Geometry check sheet. Reference: the model listing, model coordinates, mm. Coordinates: 2 decimals unless noted, no trailing zeros. Write each loop counter-clockwise with the first axis right and the second up, starting at its lowest first coordinate (ties: lowest second). Pieces come first, ordered by that corner, then holes. Notation, with made-up numbers: (65, 30.5) -> (71, 30.5) arc R9 ccw to (71, 41.5) -> close; hole circle Ø1 at (-22, 69.25). An arc over 180 degrees is marked (long way). Answer as CSV lines item,"result".
```python
from build123d import *

# Parameters (mm, degrees)
F0_W     = 292.1
F0_H     = 50.8
F1_DEPTH = 12.7
F6_D     = 4.9784
F7_W     = 2.413
F7_H     = 2.8018399096
F8_DEPTH = 292.1


with BuildPart() as f1:
    # F0 (on Top) → F1 (new body)
    with BuildSketch(Plane.XY):
        with Locations((146.05, 25.4)):
            Rectangle(F0_W, F0_H)
    extrude(amount=-F1_DEPTH)

    # F6 (through all)
    with Locations(Plane.XY):
        with Locations((6.35, 40.64), (285.75, 40.64), (285.75, 10.16), (6.35, 10.16)):
            Hole(F6_D / 2)

    # F7 (on face) → F8 (cut, through all)
    with BuildSketch(Plane.YZ.offset(292.1)):
        Polygon((3.81, -3.81), (0, -3.81), (0, -5.4102), (2.413, -5.4102), (3.81, -5.4102), align=None)
        with Locations((1.2065, -6.8111199548)):
            Rectangle(F7_W, F7_H)
        Polygon((2.413, -8.2120399096), (0, -8.2120399096), (0, -12.7), (3.81, -12.7), (3.81, -8.2120399096), align=None)
        Polygon((50.8, -5.4102), (50.8, -3.81), (46.99, -3.81), (46.99, -5.4102), (48.387, -5.4102), align=None)
        with Locations((49.5935, -6.8111199548)):
            Rectangle(F7_W, F7_H)
        Polygon((46.99, -8.2120399096), (46.99, -12.7), (50.8, -12.7), (50.8, -8.2120399096), (48.387, -8.2120399096), align=None)
    extrude(amount=-F8_DEPTH, mode=Mode.SUBTRACT)


solid = f1.part
```
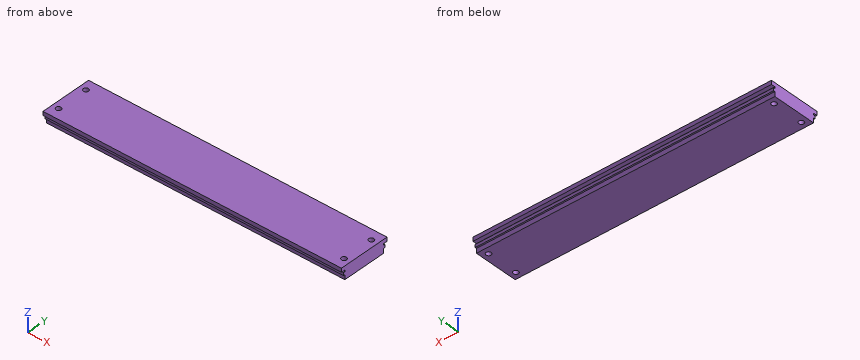
Item 1: Cross-section at B-B, the plane y = 40.64. Record the cut outline in (x, z), plus the area to 3 significant figures.
Responses:
outline,"(0, -12.7) -> (3.86, -12.7) -> (3.86, 0) -> (0, 0) -> close; (8.84, -12.7) -> (283.26, -12.7) -> (283.26, 0) -> (8.84, 0) -> close; (288.24, -12.7) -> (292.1, -12.7) -> (292.1, 0) -> (288.24, 0) -> close"
area,"3,580 mm2"
Item 2: Thickness scan on probe 1 along Y at (x, z) = (285.75, -10); probe 2 along Y at (x, z) = (285.75, -7); probe 3 along Y at (x, z) = (133, -8.75). Record the ranges inside material, lowest first.
Responses:
probe 1,"y = 3.81 to 7.67, 12.65 to 38.15, 43.13 to 46.99"
probe 2,"y = 2.41 to 7.67, 12.65 to 38.15, 43.13 to 48.39"
probe 3,"y = 3.81 to 46.99"
Item 3: Cross-section at C-C, the plane x = 285.75. Record the cut outline in (y, z).
Responses:
outline,"(0, -3.81) -> (3.81, -3.81) -> (3.81, -5.41) -> (2.41, -5.41) -> (2.41, -8.21) -> (3.81, -8.21) -> (3.81, -12.7) -> (7.67, -12.7) -> (7.67, 0) -> (0, 0) -> close; (12.65, -12.7) -> (38.15, -12.7) -> (38.15, 0) -> (12.65, 0) -> close; (43.13, -12.7) -> (46.99, -12.7) -> (46.99, -8.21) -> (48.39, -8.21) -> (48.39, -5.41) -> (46.99, -5.41) -> (46.99, -3.81) -> (50.8, -3.81) -> (50.8, 0) -> (43.13, 0) -> close"
Item 4: Cross-section at A-A, the plane z = -10.5. Record the cut outline in (x, y), plus the area to 3 significant figures.
Responses:
outline,"(0, 3.81) -> (292.1, 3.81) -> (292.1, 46.99) -> (0, 46.99) -> close; hole circle Ø4.98 at (6.35, 10.16); hole circle Ø4.98 at (6.35, 40.64); hole circle Ø4.98 at (285.75, 10.16); hole circle Ø4.98 at (285.75, 40.64)"
area,"12,500 mm2"
Item 5: Depth check by flat-ended pin: pin 1 Ø0.5 at (x, z) = (110, -5) entering from -Y; pin 2 Ø0.7 at (x, y) = (102, 47.5) entering from -Z; pin 3 Ø0.8 at (x, z) = (184.5, -4.5) entering from +Y. Enter the tip coordinate at first touch or a pass-through.
Responses:
pin 1,"stops at y = 3.81"
pin 2,"stops at z = -8.21"
pin 3,"stops at y = 46.99"
Item 6: Cross-section at D-D, the plane x = 78. Record the cut outline in (y, z), plus the area to 3 significant figures.
Responses:
outline,"(0, -3.81) -> (3.81, -3.81) -> (3.81, -5.41) -> (2.41, -5.41) -> (2.41, -8.21) -> (3.81, -8.21) -> (3.81, -12.7) -> (46.99, -12.7) -> (46.99, -8.21) -> (48.39, -8.21) -> (48.39, -5.41) -> (46.99, -5.41) -> (46.99, -3.81) -> (50.8, -3.81) -> (50.8, 0) -> (0, 0) -> close"
area,"585 mm2"
